The listing builds one solid part. Answer for the finished solid, in the listing's coordinates (mm). Face numbers are marked on the shaded views. Coordinates: 2 decimals unless noted, no trailing zeros. Loops run counter-clockwise (first coordinate to the right, second up) from the corner with the lowest first, then second, coordinate; pieces in that order, holes last. Notation, with made-up numbers: (-14.5, 57.25) - (-3.5, 57.25) arc R24 cw to (-3.5, 72.25) - close; hole circle Ø8 at (43, -1). An arc over 180 degrees is marked (long way). Put each result on its own line as item: value.
```python
from build123d import *

# Parameters (mm, degrees)
BOSS_EXTRUDE1_DEPTH = 22.225
FILLET1_R           = 0.635
SKETCH2_R           = 1.778
CUT_EXTRUDE3_DEPTH  = 8.255


with BuildPart() as part:
    # Sketch1 → Boss-Extrude1 (new body)
    with BuildSketch(Plane(origin=(0, 0, 0), x_dir=(1, 0, 0), z_dir=(0, 1, 0))):
        with BuildLine():
            Line((-1.4605, 2.286), (1.4605, 2.286))
            ThreePointArc((1.4605, 2.286), (3.7465, 0), (1.4605, -2.286))
            Line((1.4605, -2.286), (-1.4605, -2.286))
            ThreePointArc((-1.4605, -2.286), (-3.7465, 0), (-1.4605, 2.286))
        make_face()
    extrude(amount=BOSS_EXTRUDE1_DEPTH)

    # Fillet1
    fillet1_edges = [part.edges().sort_by_distance(p)[0] for p in [
        (3.7465, 22.225, 0),
        (0, 22.225, -2.286),
        (-3.7465, 22.225, 0),
        (0, 22.225, 2.286),
    ]]
    fillet(fillet1_edges, radius=FILLET1_R)

    # Sketch2 → Cut-Extrude3 (cut)
    with BuildSketch(Plane.XZ):
        Circle(SKETCH2_R)
    extrude(amount=-CUT_EXTRUDE3_DEPTH, mode=Mode.SUBTRACT)


solid = part.part
```
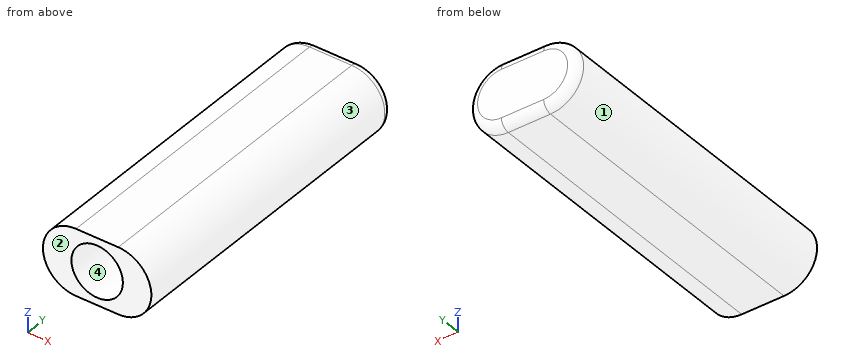
1) The part is cut by section B-B (y = 1.5). Give the vertices of the cut face in (x, z).
Found:
outline: (-1.46, -2.29) - (1.46, -2.29) arc R2.29 ccw to (1.46, 2.29) - (-1.46, 2.29) arc R2.29 ccw to start; hole circle Ø3.56 at (0, 0)
2) This flat-tipped pin is pushed along its axis until it touches: pin 1 (1 mm diameter, centred on x = -2.5, y = 18, fed in from +Z). Where does it stop, or does it pass through?
Found:
pin 1: stops at z = 2.22
3) Straight lines are drawn through the part: L1, parallel to Z at x = 0, y = 1.5; L2, parallel to Y at x = 0.75, z = 0.35 (3 decimals); L3, parallel to X at y = 16.25, z = 1.65. For each, find the intervals that lie inside material, in ascending order. Write a range as [from, to].
Found:
L1: z = [-2.29, -1.78], [1.78, 2.29]
L2: y = [8.255, 22.225]
L3: x = [-3.04, 3.04]
4) The part is cut by section C-C (x = 0). Give the vertices of the cut face in (y, z) (3 decimals).
Found:
outline: (0, -2.286) - (21.59, -2.286) arc R0.635 ccw to (22.225, -1.651) - (22.225, 1.651) arc R0.635 ccw to (21.59, 2.286) - (0, 2.286) - (0, 1.778) - (8.255, 1.778) - (8.255, -1.778) - (0, -1.778) - close
5) The part is cut by section A-A (z = 0). Give the vertices of the cut face in (x, y) (1 decimal), and give its area (3 significant figures).
Found:
outline: (-3.7, 0) - (-1.8, 0) - (-1.8, 8.3) - (1.8, 8.3) - (1.8, 0) - (3.7, 0) - (3.7, 21.6) arc R0.6 ccw to (3.1, 22.2) - (-3.1, 22.2) arc R0.6 ccw to (-3.7, 21.6) - close
area: 137 mm^2
6) For a pull along X with two mould halves and no side action, classify the marked faces 1, 2, 3 and 4 as pulls with the +X half, pulls with the -X half, needs draft (parallel to the pull), parting line crosses it, or undercut.
Found:
face 1: pulls with the -X half
face 2: needs draft
face 3: pulls with the +X half
face 4: undercut
7) The part is cut by section D-D (y = 9.5). Give the vertices of the cut face in (x, z).
Found:
outline: (-1.46, -2.29) - (1.46, -2.29) arc R2.29 ccw to (1.46, 2.29) - (-1.46, 2.29) arc R2.29 ccw to start
